Autodesk Inventor part; units mm, degrees
ref_plane "YZ Plane" through (0, 0, 0) normal (1, 0, 0) x (0, 1, 0)
ref_plane "XZ Plane" through (0, 0, 0) normal (0, 1, 0) x (-1, 0, 0)
ref_plane "XY Plane" through (0, 0, 0) normal (0, 0, 1) x (1, 0, 0)
sketch "Sketch1" plane through (0, 0, 0) normal (0, 1, 0) x (-1, 0, 0)
  circle A0 centre (0, 0) radius 14.2875
  circle A1 centre (87.63, -19.05) radius 3.3782
  circle A2 centre (87.63, 19.05) radius 3.3782
  circle A3 centre (40.64, 0) radius 14.2875
  line L0 (-19.05, 25.4) -> (93.98, 25.4)
  line L1 (93.98, 25.4) -> (93.98, -25.4)
  line L2 (93.98, -25.4) -> (-19.05, -25.4)
  line L3 (-19.05, -25.4) -> (-19.05, 25.4)
  dimension "d0" = 28.575
  dimension "d1" = 6.7564
  dimension "d2" = 6.7564
  dimension "d3" = 19.05
  dimension "d4" = 19.05
  dimension "d5" = 0
  dimension "d6" = 87.63
  dimension "d8" = 28.575
  dimension "d9" = 40.64
  dimension "d10" = 6.35
  dimension "d11" = 6.35
  dimension "d12" = 6.35
  dimension "d13" = 19.05
extrude "Extrusion1" add sketch "Sketch1" along normal blind 3.175
properties part number "Bearing Plate 2-1"
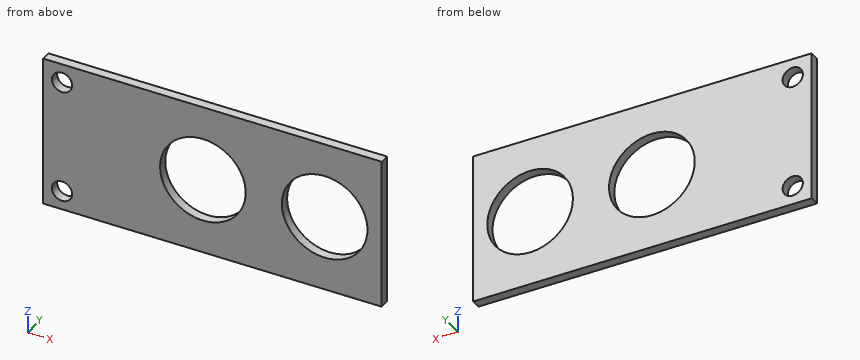
Work out the finished part from the listing and answer in its coordinate system (mm). Coordinates: 2 decimals unless noted, no trailing zeros. Loops run counter-clockwise (first coordinate to the right, second up) from the corner with the lowest first, then second, coordinate; pieces in that order, holes last. Notation, with made-up numbers: (3.25, 13.25) - (45.25, 13.25) arc R30 ccw to (45.25, 42.25) - close; hole circle Ø3 at (-31, 8.25). An arc over 180 degrees is marked (long way). Use a Markdown table: item, result.
Item 1: Find section B-B, the plane x = 0. Determine the outline of the cut face in (y, z) (1 decimal).
Evaluation:
| item | result |
|---|---|
| outline | (0, -25.4) - (3.2, -25.4) - (3.2, -14.3) - (0, -14.3) - close; (0, 14.3) - (3.2, 14.3) - (3.2, 25.4) - (0, 25.4) - close |
Item 2: Consider probe 1 along Z at (x, y) = (-87.63, 2.5); probe 2 along X at (y, z) = (2.4, 10.5); probe 3 along X at (y, z) = (0.3, -1). Determine where each line is inside the solid, lowest interval first. Write a range as from..to.
Evaluation:
| item | result |
|---|---|
| probe 1 | z = -25.4..-22.43, -15.67..15.67, 22.43..25.4 |
| probe 2 | x = -93.98..-50.33, -30.95..-9.69, 9.69..19.05 |
| probe 3 | x = -93.98..-54.89, -26.39..-14.25, 14.25..19.05 |
Item 3: Find section C-C, the plane z = 19.05. Determine the outline of the cut face in (x, y) (3 decimals), and give its area (3 significant figures).
Evaluation:
| item | result |
|---|---|
| outline | (-93.98, 0) - (-91.008, 0) - (-91.008, 3.175) - (-93.98, 3.175) - close; (-84.252, 0) - (19.05, 0) - (19.05, 3.175) - (-84.252, 3.175) - close |
| area | 337 mm2 |
Item 4: Given pin 1 Ø12 at (x, z) = (-31.5, 2.5) entering from -Y, flat-ended and moving along its own axis, determine where the tip first touches the part or whether it passes through.
Evaluation:
| item | result |
|---|---|
| pin 1 | stops at y = 0 |
Item 5: Find section A-A, the plane z = 0. State how many separate pieces and enclosed holes the cut face has, and give its area (3 significant figures).
Evaluation:
| item | result |
|---|---|
| separate pieces | 3 |
| enclosed holes | 0 |
| area | 177 mm2 |
